```python
from build123d import *

# Parameters (mm, degrees)
F1_DEPTH = 38
F2_R     = 20.15
F3_DEPTH = 26
F5_DEPTH = 91
F7_DEPTH = 34.5010000087


with BuildPart() as f1:
    # F0 (on Top) → F1 (new body)
    with BuildSketch(Plane.XY):
        with BuildLine():
            Line((8.1700673192, 21.5), (-8.1700673192, 21.5))
            ThreePointArc((-8.1700673192, 21.5), (-23, 0), (-8.1700673192, -21.5))
            Line((-8.1700673192, -21.5), (8.1700673192, -21.5))
            ThreePointArc((8.1700673192, -21.5), (23, 0), (8.1700673192, 21.5))
        make_face()
    extrude(amount=F1_DEPTH)

    # F2 (on face) → F3 (cut)
    with BuildSketch(Plane.XY.offset(38)):
        Circle(F2_R)
    extrude(amount=-F3_DEPTH, mode=Mode.SUBTRACT)

    # F4 (on face) → F5 (join)
    with BuildSketch(Plane(origin=(0, 0, 0), x_dir=(1, 0, 0), z_dir=(0, 0, -1))):
        with BuildLine():
            Line((11.4999999936, -15.7480157527), (11.5000000064, 15.7480157434))
            ThreePointArc((11.5000000064, 15.7480157434), (7.9e-09, 19.5), (-11.4999999936, 15.7480157527))
            Line((-11.4999999936, 15.7480157527), (-11.5000000064, -15.7480157434))
            ThreePointArc((-11.5000000064, -15.7480157434), (-7.9e-09, -19.5), (11.4999999936, -15.7480157527))
        make_face()
    extrude(amount=F5_DEPTH)

    # F6 (on face) → F7 (cut, through all)
    with BuildSketch(Plane(origin=(-11.5, -4.6e-09, 0), x_dir=(4e-10, -1, 0), z_dir=(-1, -4e-10, 0))):
        with BuildLine():
            ThreePointArc((-9.3808315196, -91), (-12.7417686292, -89.1480372937), (-15.748015748, -86.7630546142))
            Line((-15.748015748, -86.7630546142), (-15.748015748, -91))
            Line((-15.748015748, -91), (-9.3808315196, -91))
        make_face()
        with BuildLine():
            ThreePointArc((15.748015748, -86.7630546142), (12.7417686292, -89.1480372937), (9.3808315196, -91))
            Line((9.3808315196, -91), (15.748015748, -91))
            Line((15.748015748, -91), (15.748015748, -86.7630546142))
        make_face()
        with BuildLine():
            ThreePointArc((-15.748015748, -86.7630546142), (-21.1092913453, -79.1322406285), (-23, -70))
            Line((-23, -70), (-29.5417029411, -96.2313264608))
            Line((-29.5417029411, -96.2313264608), (26.6386214644, -96.2313264608))
            Line((26.6386214644, -96.2313264608), (23, -70))
            ThreePointArc((23, -70), (21.1092913453, -79.1322406285), (15.748015748, -86.7630546142))
            Line((15.748015748, -86.7630546142), (15.748015748, -91))
            Line((15.748015748, -91), (9.3808315196, -91))
            ThreePointArc((9.3808315196, -91), (0, -93), (-9.3808315196, -91))
            Line((-9.3808315196, -91), (-15.748015748, -91))
            Line((-15.748015748, -91), (-15.748015748, -86.7630546142))
        make_face()
    extrude(amount=-F7_DEPTH, mode=Mode.SUBTRACT)


solid = f1.part
```
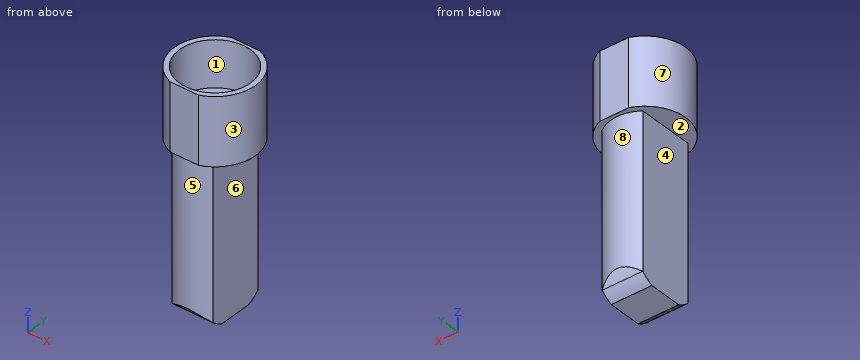
Verification items for the finished model (mm, model axes). Face numbers are marked on the shaded views. A direction names the side the tool comes from. Round coordinates to 2 decimals unless told otherwise and drop trailing zeros. Write each loop counter-clockwise with the first axis right and the second up, starting at its lowest first coordinate (ties: lowest second). Pieces come first, ordered by that corner, then holes. Notation, with made-up numbers: (-36, 11) -> (17, 11) arc R17 cw to (17, 27) -> close; hole circle Ø8 at (-14.75, -25.75). An arc over 180 degrees is marked (long way). Write each question's results on one line, items separated by ' | '. Start each with the question number.
1. Depth check by flat-ended pin: P1, Ø9.5, axis at y = -2.5, z = -25.5, coming from the -X side; P2, Ø3, axis at y = 8.5, z = -65, coming from the +X side; P3, Ø10, axis at y = 1, z = 19, coming from the -X side. Enter the tip coordinate at first touch or a pass-through.
2. Material ranges on probe 1 along Y at (x, z) = (0, 28.5); probe 2 along Z at (x, y) = (10, -9); probe 3 along Z at (x, y) = (15, -8.5), recorded low to high. Write a range as from..to.
3. Set-up check for the marked faces 4, 5, 6, 7 and 8: record each of +Z, -Z, +X, -X, +Y, -Y from which the full face is reachable in a straight line by a thin tool's end or side.
4. Draft check along X on the marked faces 1, 2 and 3. Enter one of: +X half, -X half, draft (parallel to the pull), parting line (faces both ways), or undercut.
5. Cross-section at D-D (x = 0). Enter the section's corners in (y, z).
6. Cross-section at B-B (x = -16). Enter the section's corners in (y, z).
7. Cross-section at A-A (y = 0). Enter the section's corners in (x, z), then the cut area to 3 significant figures.
8. Cross-section at C-C (z = -60.5). Enter the section's corners in (x, y), then the cut area to 3 significant figures.
Solutions:
1) P1: stops at x = -11.5 | P2: stops at x = 11.5 | P3: stops at x = -23
2) probe 1: y = -21.5..-20.15, 20.15..21.5 | probe 2: z = -91..12 | probe 3: z = 0..12
3) face 4: -Z, -X, +Y, -Y | face 5: -Z, -Y | face 6: -Z, +X, +Y, -Y | face 7: +Z, -Z, -X | face 8: -Z, +Y
4) face 1: undercut | face 2: draft | face 3: +X half
5) outline: (-21.5, 0) -> (-19.5, 0) -> (-19.5, -82.2) arc R23 ccw to (-9.38, -91) -> (9.38, -91) arc R23 ccw to (19.5, -82.2) -> (19.5, 0) -> (21.5, 0) -> (21.5, 38) -> (20.15, 38) -> (20.15, 12) -> (-20.15, 12) -> (-20.15, 38) -> (-21.5, 38) -> close
6) outline: (-16.52, 0) -> (16.52, 0) -> (16.52, 38) -> (12.25, 38) -> (12.25, 12) -> (-12.25, 12) -> (-12.25, 38) -> (-16.52, 38) -> close
7) outline: (-23, 0) -> (-11.5, 0) -> (-11.5, -91) -> (11.5, -91) -> (11.5, 0) -> (23, 0) -> (23, 38) -> (20.15, 38) -> (20.15, 12) -> (-20.15, 12) -> (-20.15, 38) -> (-23, 38) -> close | area: 2,790 mm2
8) outline: (-11.5, -15.75) arc R19.5 ccw to (11.5, -15.75) -> (11.5, 15.75) arc R19.5 ccw to (-11.5, 15.75) -> close | area: 842 mm2
